Verification items for the finished model (mm, model axes). A direction names the side the tool comes from. Round coordinates to 2 decimals unless told otherwise and drop trailing zeros. Loops run counter-clockwise (first coordinate to the right, second up) from the corner with the lowest first, then second, coordinate; pieces in that order, holes last. Notation, with made-up numbers: (-21, 11) -> (8, 11) arc R12 ccw to (8, 22) -> close; hole circle Ø6 at (-10.5, -28.75). An arc over 180 degrees is marked (long way). Write item = value, one per line.
```python
from build123d import *

# Parameters (mm, degrees)
SKETCH_1_W      = 600
SKETCH_1_H      = 700
EXTRUDE_1_DEPTH = 140
SHELL_1_T       = -1
HOLE_WIZARD_1_D = 57


with BuildPart() as part:
    # 草图1 → 凸台-拉伸1 (new, symmetric)
    with BuildSketch(Plane.XY):
        Rectangle(SKETCH_1_W, SKETCH_1_H)
    extrude(amount=EXTRUDE_1_DEPTH, both=True)

    # 抽壳1
    shell_1_openings = [part.faces().sort_by_distance(p)[0] for p in [
        (0, -350, 0),
    ]]
    offset(amount=SHELL_1_T, openings=shell_1_openings, kind=Kind.INTERSECTION)

    # 孔1 (through all)
    with Locations(Plane(origin=(0, 350, 0), x_dir=(1, 0, 0), z_dir=(0, 1, 0))):
        with Locations((0, 79)):
            Hole(HOLE_WIZARD_1_D / 2)


solid = part.part
```
(1) Draft check along Z on faces 1 (the face through (-4, 5, 140)), 2 (the face through (-4, 350, 2)), 3 (the face through (-4, 349, 2)). Enter one of: released by +Z, released by -Z, zero draft, split by the parting line, or undercut.
Filled sheet:
face_1 = released by +Z
face_2 = zero draft
face_3 = undercut
(2) Set-up check for faces 4 (the face through (299, -5, 2)), 5 (the face through (-4, 5, -140)): record each of +Z, -Z, +X, -X, +Y, -Y from which the full face is reachable in a straight line by a thin tool's end or side.
Filled sheet:
face_4 = -Y
face_5 = -Z, +X, -X, +Y, -Y
(3) Material ranges on probe 1 along Z at (x, y) = (-71.5, -254); probe 2 along X at (y, z) = (349.45, -79); probe 3 along X at (y, z) = (-234.5, 6.5), recorded low to high. Write a range as from..to.
Filled sheet:
probe_1 = -140..-139, 139..140
probe_2 = -300..-28.5, 28.5..300
probe_3 = -300..-299, 299..300
(4) Sectioned sample at D-D, the plane x = 80. Record the cut outline in (y, z).
Filled sheet:
outline = (-350, -140) -> (350, -140) -> (350, 140) -> (-350, 140) -> (-350, 139) -> (349, 139) -> (349, -139) -> (-350, -139) -> close
(5) Sectioned sample at A-A, the plane y = 224. Record the cut outline in (x, z).
Filled sheet:
outline = (-300, -140) -> (300, -140) -> (300, 140) -> (-300, 140) -> close; hole (-299, -139) -> (299, -139) -> (299, 139) -> (-299, 139) -> close
(6) Sectioned sample at B-B, the plane x = 0. Record the cut outline in (y, z).
Filled sheet:
outline = (-350, -140) -> (350, -140) -> (350, -107.5) -> (349, -107.5) -> (349, -139) -> (-350, -139) -> close; (-350, 139) -> (349, 139) -> (349, -50.5) -> (350, -50.5) -> (350, 140) -> (-350, 140) -> close
(7) Go/stop test with a flat-tipped pin: pin 1 Ø6 at (x, z) = (-130.5, -85.5) entering from -Y. Record where the tip stops, or that it passes through.
Filled sheet:
pin_1 = 349
(8) Sectioned sample at C-C, the plane z = -79. Record the cut outline in (x, y), and give its area (3 significant figures).
Filled sheet:
outline = (-300, -350) -> (-299, -350) -> (-299, 349) -> (-28.5, 349) -> (-28.5, 350) -> (-300, 350) -> close; (28.5, 349) -> (299, 349) -> (299, -350) -> (300, -350) -> (300, 350) -> (28.5, 350) -> close
area = 1,940 mm2
